```python
from build123d import *

# Parameters (mm, degrees)
EXTRUDE1_DEPTH  = 2.54
EXTRUDE2_DEPTH  = 3.54
EXTRUDE3_DEPTH  = 3.54
FILLET1_R       = 0.762
SKETCH6_R       = 1.016
EXTRUDE6_DEPTH  = 3.54
EXTRUDE9_DEPTH  = 0.508
EXTRUDE10_DEPTH = 0.508


with BuildPart() as part:
    # Sketch1 → Extrude1 (new body)
    with BuildSketch(Plane.XY):
        with BuildLine():
            Line((-3.682902029, 0.407863494), (-2.38382675, 0.407863494))
            ThreePointArc((-2.38382675, 0.407863494), (-2.229201347, 0.460351745), (-2.13848159, 0.596123456))
            Line((-2.13848159, 0.596123456), (-1.280622225, 3.797698194))
            ThreePointArc((-1.280622225, 3.797698194), (-1.179315691, 3.971165577), (-1.003864933, 4.068996952))
            ThreePointArc((-1.003864933, 4.068996952), (0, 4.191), (1.003864933, 4.068996952))
            ThreePointArc((1.003864933, 4.068996952), (1.179315691, 3.971165577), (1.280622225, 3.797698194))
            Line((1.280622225, 3.797698194), (2.13848159, 0.596123456))
            ThreePointArc((2.13848159, 0.596123456), (2.229201347, 0.460351745), (2.38382675, 0.407863494))
            Line((2.38382675, 0.407863494), (3.682902029, 0.407863494))
            ThreePointArc((3.682902029, 0.407863494), (3.951325396, 0.297251911), (4.063891894, 0.029642476))
            ThreePointArc((4.063891894, 0.029642476), (3.409731918, -2.2112947), (1.63048159, -3.722583214))
            ThreePointArc((1.63048159, -3.722583214), (1.594432949, -3.838601921), (1.498982382, -3.913761978))
            ThreePointArc((1.498982382, -3.913761978), (0, -4.191), (-1.498982382, -3.913761978))
            ThreePointArc((-1.498982382, -3.913761978), (-1.594432949, -3.838601921), (-1.63048159, -3.722583214))
            ThreePointArc((-1.63048159, -3.722583214), (-3.409731918, -2.2112947), (-4.063891894, 0.029642476))
            ThreePointArc((-4.063891894, 0.029642476), (-3.951325396, 0.297251911), (-3.682902029, 0.407863494))
        make_face()
    extrude(amount=EXTRUDE1_DEPTH)

    # Sketch2 → Extrude2 (cut, through all)
    with BuildSketch(Plane.XY.offset(2.54)):
        with BuildLine():
            Line((-2.38382675, 0.407863494), (-3.682902029, 0.407863494))
            ThreePointArc((-3.682902029, 0.407863494), (-3.951325396, 0.297251911), (-4.063891894, 0.029642476))
            ThreePointArc((-4.063891894, 0.029642476), (-4.047838367, -0.362078102), (-3.994114692, -0.750429096))
            Line((-3.994114692, -0.750429096), (-2.356119493, 0.102257234))
            ThreePointArc((-2.356119493, 0.102257234), (-2.275312982, 0.168573423), (-2.228058481, 0.261817948))
            Line((-2.228058481, 0.261817948), (-2.13848159, 0.596123456))
            ThreePointArc((-2.13848159, 0.596123456), (-2.229201347, 0.460351745), (-2.38382675, 0.407863494))
        make_face()
    extrude(amount=-EXTRUDE2_DEPTH, mode=Mode.SUBTRACT)

    # Sketch3 → Extrude3 (cut, through all)
    with BuildSketch(Plane.XY.offset(2.54)):
        with BuildLine():
            Line((3.682902029, 0.407863494), (2.38382675, 0.407863494))
            ThreePointArc((2.38382675, 0.407863494), (2.229201347, 0.460351745), (2.13848159, 0.596123456))
            Line((2.13848159, 0.596123456), (2.228058481, 0.261817948))
            ThreePointArc((2.228058481, 0.261817948), (2.275312982, 0.168573423), (2.356119493, 0.102257234))
            Line((2.356119493, 0.102257234), (3.994114692, -0.750429096))
            ThreePointArc((3.994114692, -0.750429096), (4.047838367, -0.362078102), (4.063891894, 0.029642476))
            ThreePointArc((4.063891894, 0.029642476), (3.951325396, 0.297251911), (3.682902029, 0.407863494))
        make_face()
    extrude(amount=-EXTRUDE3_DEPTH, mode=Mode.SUBTRACT)

    # Fillet1
    fillet1_edges = [part.edges().sort_by_distance(p)[0] for p in [
        (-3.994114692, -0.750429096, 1.27),
        (3.994114692, -0.750429096, 1.27),
    ]]
    fillet(fillet1_edges, radius=FILLET1_R)

    # Sketch6 → Extrude6 (cut, through all)
    with BuildSketch(Plane.XY.offset(2.54)):
        Circle(SKETCH6_R)
    extrude(amount=-EXTRUDE6_DEPTH, mode=Mode.SUBTRACT)

    # Sketch11 → Cut-Revolve1 (revolve, cut)
    with BuildSketch(Plane(origin=(0, 0, 0), x_dir=(1, 0, 0), z_dir=(0, 1, 0))):
        Polygon((0, -2.54), (1.524, -2.54), (0.508, -1.524), (0.508, -1.016), (1.524, 0), (0, 0), align=None)
    revolve(axis=Axis((0, 0, 0), (0, 0, 1)), mode=Mode.SUBTRACT)

    # Sketch9 → Extrude9 (cut)
    with BuildSketch(Plane(origin=(0, 0, 0), x_dir=(-1, 0, 0), z_dir=(0, 0, -1))):
        with BuildLine():
            Line((-0.381, 3.429), (0.381, 3.429))
            ThreePointArc((0.381, 3.429), (0.650407684, 3.317407684), (0.762, 3.048))
            Line((0.762, 3.048), (0.762, 0.672020833))
            Line((0.762, 0.672020833), (-0.762, 0.672020833))
            Line((-0.762, 0.672020833), (-0.762, 3.048))
            ThreePointArc((-0.762, 3.048), (-0.650407684, 3.317407684), (-0.381, 3.429))
        make_face()
    extrude(amount=-EXTRUDE9_DEPTH, mode=Mode.SUBTRACT)

    # Sketch10 → Extrude10 (cut)
    with BuildSketch(Plane.XY.offset(2.54)):
        with BuildLine():
            Line((-0.381, 3.429), (0.381, 3.429))
            ThreePointArc((0.381, 3.429), (0.650407684, 3.317407684), (0.762, 3.048))
            Line((0.762, 3.048), (0.762, 0.672020833))
            Line((0.762, 0.672020833), (-0.762, 0.672020833))
            Line((-0.762, 0.672020833), (-0.762, 3.048))
            ThreePointArc((-0.762, 3.048), (-0.650407684, 3.317407684), (-0.381, 3.429))
        make_face()
    extrude(amount=-EXTRUDE10_DEPTH, mode=Mode.SUBTRACT)


solid = part.part
```
Geometry: final body of the model. Coordinates: model frame, mm. A direction names the side the tool comes from. Coordinates: 2 decimals unless noted, no trailing zeros. Order: outer loops, then holes, each group sorted by start corner. A loop starts at its lowest first (then second) coordinate and runs counter-clockwise, first axis right, second up. Notation, with made-up numbers: (13.5, -29) - (25.5, -29) arc R20 ccw to (25.5, 10) - close; hole circle Ø5 at (71.5, 20.25). An arc over 180 degrees is marked (long way). Return JSON: item names as keys, results as strings. Group by question number.
1. Cut plane B-B (z = 1.35). Output: boundary loops of the cut face in (x, y), plus the area to 3 significant figures.
2. Pin query (flat end, axial travel): pin 1 (1.6 mm diameter, centred on x = 0, y = 0, fed in from -Z); pin 2 (1.7 mm diameter, centred on x = 0, y = 1.5, fed in from +Z). Return the tip coordinate at first contact, or that it passes through.
3. Cut plane D-D (y = 2). Output: boundary loops of the cut face in (x, z).
4. Cut plane C-C (y = 0). Output: boundary loops of the cut face in (x, z).
5. Cut plane A-A (x = 0). Output: boundary loops of the cut face in (y, z), plus the area to 3 significant figures.
6. Set-up query: faces 5 (the face through (3.811, -0.876, 1.252)), 6 (the face through (0, 2, 0.508)). Return all of +Z, -Z, +X, -X, +Y, -Y with unobstructed straight access to the full face (end or side cutting, diameter ignored); none if empty.
7. Pull-direction query (Y, two-part tool) for faces 1 (the face through (0.02, -4.19, 1.25)), 2 (the face through (2.9, -0.18, 1.29)), 3 (the face through (0, 2, 2.032)), 4 (the face through (-3.806, -0.861, 1.252)); classes: pulls with the +Y half, pulls with the -Y half, needs draft (parallel to the pull), parting line crosses it, or undercut.
8. Material intervals for line 1 along Y through (x, z) = (0, 1.65); line 2 along X through (y, z) = (0, 0.9); line 3 along X through (y, z) = (2.5, 0.4), sorted ascending. Write a range as [from, to].
Resolved:
{
 "1": {"outline": "(-3.81, -1.41) arc R4.06 ccw to (-1.63, -3.72) arc R0.2 ccw to (-1.5, -3.91) arc R4.19 ccw to (1.5, -3.91) arc R0.2 ccw to (1.63, -3.72) arc R4.06 ccw to (3.81, -1.41) arc R0.76 ccw to (3.45, -0.47) - (2.36, 0.1) arc R0.25 cw to (2.23, 0.26) - (1.28, 3.8) arc R0.38 ccw to (1, 4.07) arc R4.19 ccw to (-1, 4.07) arc R0.38 ccw to (-1.28, 3.8) - (-2.23, 0.26) arc R0.25 cw to (-2.36, 0.1) - (-3.45, -0.47) arc R0.76 ccw to start; hole circle Ø2.03 at (0, 0)", "area": "36.3 mm²"},
 "2": {"pin 1": "passes through", "pin 2": "stops at z = 2.54"},
 "3": {"outline": "(-1.76, 0) - (-0.76, 0) - (-0.76, 0.51) - (0.76, 0.51) - (0.76, 0) - (1.76, 0) - (1.76, 2.54) - (0.76, 2.54) - (0.76, 2.03) - (-0.76, 2.03) - (-0.76, 2.54) - (-1.76, 2.54) - close"},
 "4": {"outline": "(-2.55, 0) - (-1.52, 0) - (-1.02, 0.51) - (-1.02, 2.03) - (-1.52, 2.54) - (-2.55, 2.54) - close; (1.02, 0.51) - (1.52, 0) - (2.55, 0) - (2.55, 2.54) - (1.52, 2.54) - (1.02, 2.03) - close"},
 "5": {"outline": "(-4.19, 0) - (-1.52, 0) - (-1.02, 0.51) - (-1.02, 2.03) - (-1.52, 2.54) - (-4.19, 2.54) - close; (1.02, 0.51) - (3.43, 0.51) - (3.43, 0) - (4.19, 0) - (4.19, 2.54) - (3.43, 2.54) - (3.43, 2.03) - (1.02, 2.03) - close", "area": "13.4 mm²"},
 "6": {"face 5": "+Z, -Z, +X", "face 6": "-Z"},
 "7": {"face 1": "pulls with the -Y half", "face 2": "pulls with the +Y half", "face 3": "undercut", "face 4": "parting line crosses it"},
 "8": {"line 1": "y = [-4.19, -1.02], [1.02, 4.19]", "line 2": "x = [-2.55, -1.02], [1.02, 2.55]", "line 3": "x = [-1.63, -0.76], [0.76, 1.63]"}
}
